```python
from build123d import *

# Parameters (mm, degrees)
BOSS_EXTRUDE6_DEPTH = 9.955320875


with BuildPart() as part:
    # Sketch1 → Boss-Extrude6 (new body)
    with BuildSketch(Plane.XY):
        with BuildLine():
            Line((-51.139816159, 9.78390553), (-41.19267445, 9.782935976))
            ThreePointArc((-41.19267445, 9.782935976), (-40.46615036, 12.469308879), (-39.564350519, 15.102024906))
            ThreePointArc((-39.564350519, 15.102024906), (-31.695161559, 17.596213673), (-33.764455715, 25.587654982))
            ThreePointArc((-33.764455715, 25.587654982), (-0.032994911, 42.351160958), (33.670827225, 25.532155221))
            ThreePointArc((33.670827225, 25.532155221), (31.692118999, 17.608927269), (39.44794108, 15.051574876))
            ThreePointArc((39.44794108, 15.051574876), (40.338215404, 12.444464282), (41.056685691, 9.784875128))
            Line((41.056685691, 9.784875128), (51.004283921, 9.78390553))
            ThreePointArc((51.004283921, 9.78390553), (-0.067766119, 52.083843354), (-51.139816159, 9.78390553))
        make_face()
    extrude(amount=BOSS_EXTRUDE6_DEPTH)


solid = part.part
```
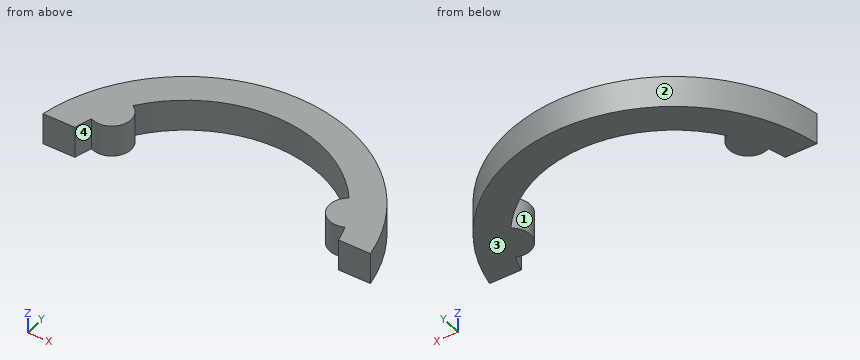
Geometry check sheet. Reference: the model listing, model coordinates, mm. Face numbers are marked on the shaded views. Coordinates: 2 decimals unless noted, no trailing zeros. Write each loop counter-clockwise with the first axis right and the second up, starting at its lowest first coordinate (ties: lowest second). Pieces come first, ordered by that corner, then holes. Notation, with made-up numbers: M 12.25,59 L 41.25,59 A17 ccw 41.25,74 Z; hole C -19,58 d3. An arc over 180 degrees is marked long. Use one line per item in the form item = value. Start each with the question number.
1) Section check A-A on y = 28.5. Enter the section's corners in (x, z), and give its area (3 significant figures).
2) Go/stop test with flat-tipped pins: pin 1 Ø3 at (y, z) = (31, 4.5) entering from +X; pin 2 Ø2 at (x, z) = (15, 4.5) entering from +Y. Record where each tip stops, or that it passes through.
3) Section check D-D on x = 42. Enter the section's corners in (y, z), and give its area (3 significant figures).
4) Section check B-B on z = 1. Enter the section's corners in (x, y), and give its area (3 significant figures).
5) Section check C-C on y = 16. Enter the section's corners in (x, z).
6) Thickness scan on probe 1 along X at (y, z) = (22.5, 3.5); probe 2 along X at (y, z) = (38, 2.5); probe 3 along Y at (x, z) = (7.5, 2). Record the ranges inside material, lowest first. Write a range as from..to.
7) Release check for a two-part mould opening along Y. For the marked faces 1, 2, 3 and 4 record: pulls with the +Y half, pulls with the -Y half, needs draft (parallel to the pull), parting line crosses it, or undercut.
Responses:
q1.outline = M -43.61,0 L -31.35,0 L -31.35,9.96 L -43.61,9.96 Z; M 31.21,0 L 43.47,0 L 43.47,9.96 L 31.21,9.96 Z
q1.area = 244 mm2
q2.pin_1 = 42.8
q2.pin_2 = 50.14
q3.outline = M 9.78,0 L 30.64,0 L 30.64,9.96 L 9.78,9.96 Z
q3.area = 208 mm2
q4.outline = M -51.14,9.78 L -41.19,9.78 A42.25 cw -39.56,15.1 A6 ccw -33.76,25.59 A42.25 cw 33.67,25.53 A6 ccw 39.45,15.05 A42.25 cw 41.06,9.78 L 51,9.78 A51.98 ccw Z
q4.area = 1,360 mm2
q5.outline = M -49.56,0 L -32.98,0 L -32.98,9.96 L -49.56,9.96 Z; M 32.98,0 L 49.42,0 L 49.42,9.96 L 32.98,9.96 Z
q6.probe_1 = -46.98..-31.29, 31.29..46.84
q6.probe_2 = -35.65..-18.74, 18.61..35.51
q6.probe_3 = 41.67..51.53
q7.face_1 = undercut
q7.face_2 = pulls with the +Y half
q7.face_3 = needs draft
q7.face_4 = pulls with the -Y half
